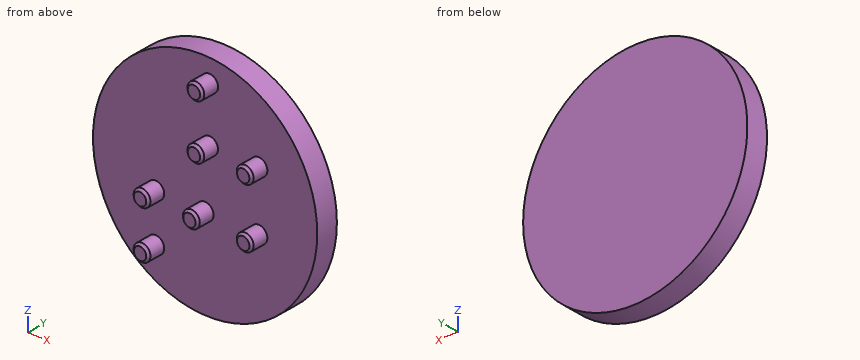
```python
from build123d import *

# Parameters (mm, degrees)
F0_R     = 50
F1_DEPTH = 10
F2_R     = 3.75
F3_DEPTH = 8
F4_SIZE  = 1


with BuildPart() as f1:
    # F0 (on Front) → F1 (new body)
    with BuildSketch(Plane.XZ):
        Circle(F0_R)
    extrude(amount=F1_DEPTH)

    # F2 (on face) → F3 (join)
    with BuildSketch(Plane.XZ.offset(10)):
        with Locations((2, 40)):
            Circle(F2_R)
        with Locations((2, 16)):
            Circle(F2_R)
        with Locations((24, 16)):
            Circle(F2_R)
        with Locations((24, -10)):
            Circle(F2_R)
        with Locations((0, -10)):
            Circle(F2_R)
        with Locations((-22, -10)):
            Circle(F2_R)
        with Locations((-22, -31)):
            Circle(F2_R)
    extrude(amount=F3_DEPTH)

    # F4
    f4_edges = [f1.edges().sort_by_distance(p)[0] for p in [
        (-1.75, -18, 40),
        (-1.75, -18, 16),
        (20.25, -18, 16),
        (20.25, -18, -10),
        (-3.75, -18, -10),
        (-25.75, -18, -10),
        (-25.75, -18, -31),
    ]]
    chamfer(f4_edges, length=F4_SIZE)


solid = f1.part
```
Geometry: final body of the model. Coordinates: model frame, mm. Coordinates: 2 decimals unless noted, no trailing zeros. Order: outer loops, then holes, each group sorted by start corner. A loop starts at its lowest first (then second) coordinate and runs counter-clockwise, first axis right, second up. Notation, with made-up numbers: M 28,-15.75 L 70,-15.75 A30 ccw 70,12.25 Z; hole C -32,28.25 d9. An arc over 180 degrees is marked long. Answer in a Markdown table with one row per item. Add a question column.
Q1. Section query A-A on z = -31. Return the cut outline in (x, y), and give its area (3 significant figures).
Q2. Section query C-C on y = -7.25. Return the cut outline in (x, z).
Q3. Section query B-B on x = 24. Return the cut outline in (y, z), and give its area (3 significant figures).
Q4. Section query D-D on z = 16. Return the cut outline in (x, y).
Q5. Line query: L1, parallel to Y at x = 10, z = 0; L2, parallel to X at y = -15, z = -8; L3, parallel to Z at x = -21.5, y = -13.75. Output: solid intervals per line, ascending.
Q6. Contact query for flat-ended pins moving along their axis: P1, Ø3, axis at y = -3.5, z = 38.5, coming from the +X side; P2, Ø8, axis at x = -13.5, y = -3.5, coming from the +Z side; P3, Ø3, axis at y = -3, z = -24, coming from the +X side. Output: stop coordinate, or through.
Completed:
| question | item | result |
|---|---|---|
| 1 | outline | M -39.23,-10 L -25.75,-10 L -25.75,-17 L -24.75,-18 L -19.25,-18 L -18.25,-17 L -18.25,-10 L 39.23,-10 L 39.23,0 L -39.23,0 Z |
| 1 | area | 844 mm2 |
| 2 | outline | C 0,0 d100 |
| 3 | outline | M -18,-12.75 L -17,-13.75 L -10,-13.75 L -10,-43.86 L 0,-43.86 L 0,43.86 L -10,43.86 L -10,19.75 L -17,19.75 L -18,18.75 L -18,13.25 L -17,12.25 L -10,12.25 L -10,-6.25 L -17,-6.25 L -18,-7.25 Z |
| 3 | area | 995 mm2 |
| 4 | outline | M -47.37,-10 L -1.75,-10 L -1.75,-17 L -0.75,-18 L 4.75,-18 L 5.75,-17 L 5.75,-10 L 20.25,-10 L 20.25,-17 L 21.25,-18 L 26.75,-18 L 27.75,-17 L 27.75,-10 L 47.37,-10 L 47.37,0 L -47.37,0 Z |
| 5 | L1 | y = -10 to 0 |
| 5 | L2 | x = -25.17 to -18.83, -3.17 to 3.17, 20.83 to 27.17 |
| 5 | L3 | z = -34.72 to -27.28, -13.72 to -6.28 |
| 6 | P1 | stops at x = 33.63 |
| 6 | P2 | stops at z = 49.09 |
| 6 | P3 | stops at x = 44.65 |
